```python
from build123d import *

# Parameters (mm, degrees)
SKETCH2_R                = 11.43
BOSS_EXTRUDE1_DEPTH      = 5.08
BOSS_EXTRUDE2_DEPTH      = 5.08
SKETCH4_R                = 4.318
SKETCH4_R_2              = 2.032
CUT_EXTRUDE1_DEPTH       = 5.08
CIRPATTERN1_COUNT        = 4
BOSS_EXTRUDE3_DEPTH      = 38.1
BOSS_EXTRUDE3_DEPTH_BACK = 40.64
SKETCH9_R                = 11.43
BOSS_EXTRUDE4_DEPTH      = 6.35


with BuildPart() as part:
    # Sketch2 → Boss-Extrude1 (new body)
    with BuildSketch(Plane.XY):
        Circle(SKETCH2_R)
    extrude(amount=BOSS_EXTRUDE1_DEPTH)

    # Sketch7 → Boss-Extrude2 (add)
    with BuildSketch(Plane(origin=(0, 0, 0), x_dir=(-1, 0, 0), z_dir=(0, 0, -1))):
        with BuildLine():
            Line((0, 11.43), (32.334928423, 11.43))
            ThreePointArc((32.334928423, 11.43), (43.764928423, 0), (32.334928423, -11.43))
            Line((32.334928423, -11.43), (0, -11.43))
            Line((0, -11.43), (0, 11.43))
        make_face()
    extrude(amount=-BOSS_EXTRUDE2_DEPTH)

    # Sketch4 → Cut-Extrude1 (cut)
    with BuildSketch(Plane(origin=(0, 0, 0), x_dir=(-1, 0, 0), z_dir=(0, 0, -1))):
        Circle(SKETCH4_R)
        with Locations((0, -8.001)):
            Circle(SKETCH4_R_2)
    cut_extrude1 = extrude(amount=-CUT_EXTRUDE1_DEPTH, mode=Mode.SUBTRACT)

    # CirPattern1: Cut-Extrude1 ×4 about axis
    cirpattern1_axis = Axis((0, 0, 0), (0, 0, 1))
    for i in range(1, CIRPATTERN1_COUNT):
        add(cut_extrude1.rotate(cirpattern1_axis, i * 360 / CIRPATTERN1_COUNT), mode=Mode.SUBTRACT)

    # Sketch9 → Boss-Extrude3 (add, two sides: drawn at the far end of the back side and taken through both)
    with BuildSketch(Plane.XY.offset(5.08).offset(-BOSS_EXTRUDE3_DEPTH_BACK)):
        with Locations((-32.334928423, 0)):
            Circle(SKETCH9_R)
    extrude(amount=BOSS_EXTRUDE3_DEPTH + BOSS_EXTRUDE3_DEPTH_BACK)

    # Sketch10 → Boss-Extrude4 (add)
    with BuildSketch(Plane.XY.offset(-31.75)):
        with BuildLine():
            Line((-37.028733454, -72.582202646), (-43.258278065, -30.219589225))
            Line((-43.258278065, -30.219589225), (-20.904928423, 0))
            Line((-20.904928423, 0), (-32.171436877, 0.015474968))
            Line((-32.171436877, 0.015474968), (-39.730825163, 0.025858069))
            Line((-39.730825163, 0.025858069), (-53.950343023, -30.219589225))
            Line((-53.950343023, -30.219589225), (-53.950343023, -58.308345581))
            Line((-53.950343023, -58.308345581), (-43.258278065, -84.842076202))
            Line((-43.258278065, -84.842076202), (-24.756596451, -88.874141931))
            ThreePointArc((-24.756596451, -88.874141931), (-19.207535115, -84.404142538), (-24.756596451, -79.934143145))
            Line((-24.756596451, -79.934143145), (-37.028733454, -72.582202646))
        make_face()
    boss_extrude4 = extrude(amount=BOSS_EXTRUDE4_DEPTH)

    # Mirror1: Boss-Extrude4 across plane
    add(boss_extrude4.mirror(Plane.XY))


solid = part.part
```
Read the model definition and answer for the solid it produces. Units are mm, in the model's axes. A direction names the side the tool comes from. Coordinates: 2 decimals unless noted, no trailing zeros. Loops run counter-clockwise (first coordinate to the right, second up) from the corner with the lowest first, then second, coordinate; pieces in that order, holes last.
(1) The mould has two halves that part along Z. Classify faces 3 (the face through (-19.21, -84.52, -28.62)), 4 (the face through (-41, -56, 31.75)), 5 (the face through (-41, -56, 25.4)): released by +Z, released by -Z, zero draft, split by the parting line, or undercut.
Solution:
face 3: zero draft
face 4: released by +Z
face 5: undercut
(2) The part is cut by section B-B (y = -26). Determine the outline of the cut face in (x, z), and give its area (3 significant figures).
Solution:
outline: (-51.97, -31.75) - (-40.14, -31.75) - (-40.14, -25.4) - (-51.97, -25.4) - close; (-51.97, 25.4) - (-40.14, 25.4) - (-40.14, 31.75) - (-51.97, 31.75) - close
area: 150 mm2
(3) The part is cut by section A-A (y = 0). Determine the outline of the cut face in (x, z).
Solution:
outline: (-43.76, -35.56) - (-20.9, -35.56) - (-20.9, 0) - (-10.03, 0) - (-10.03, 5.08) - (-20.9, 5.08) - (-20.9, 43.18) - (-43.76, 43.18) - close; (-5.97, 0) - (-4.32, 0) - (-4.32, 5.08) - (-5.97, 5.08) - close; (4.32, 0) - (5.97, 0) - (5.97, 5.08) - (4.32, 5.08) - close; (10.03, 0) - (11.43, 0) - (11.43, 5.08) - (10.03, 5.08) - close
(4) A tool of negligible diameter and unlimited length cuts with its end or side. For faces 1 (the face through (-40.1, -51.7, 28.6)), 2 (the face through (-34.14, -86.83, -28.62)), from which of +Z, -Z, +X, -X, +Y, -Y can it reach the whole face along a straight path? Write none if from no direction.
Solution:
face 1: +Z, -Z, +X
face 2: +Z, -Z, -X, -Y
(5) The part is cut by section D-D (x = -15). Determine the outline of the cut face in (y, z).
Solution:
outline: (-11.43, 0) - (11.43, 0) - (11.43, 5.08) - (-11.43, 5.08) - close
(6) Flat-ended cylindrical pins translate along their axes: pin 1 Ø11 at (x, y) = (0, 0) entering from -Z; pin 2 Ø6.5 at (x, y) = (8.001, 0) entering from +Z; pin 3 Ø17.5 at (x, y) = (-42, -31.5) entering from -Z. Find the tip coordinate at first contact, or state that the pin passes through.
Solution:
pin 1: stops at z = 0
pin 2: stops at z = 5.08
pin 3: stops at z = -31.75
(7) The part is cut by section C-C (z = 3.5). Determine the outline of the cut face in (x, y).
Solution:
outline: (-32.33, -11.43) - (0, -11.43) arc R11.43 ccw to (0, 11.43) - (-32.33, 11.43) arc R11.43 ccw to start; hole circle Ø4.06 at (-8, 0); hole circle Ø8.64 at (0, 0); hole circle Ø4.06 at (0, -8); hole circle Ø4.06 at (0, 8); hole circle Ø4.06 at (8, 0)
(8) Consider line 1 along Y through (x, z) = (0, 1); line 2 along Z through (x, y) = (-41, -73); line 3 along Y through (x, z) = (-37, 30.5). Determine where each line is inside the solid, lowest interval first.
Solution:
line 1: y = -11.43 to -10.03, -5.97 to -4.32, 4.32 to 5.97, 10.03 to 11.43
line 2: z = -31.75 to -25.4, 25.4 to 31.75
line 3: y = -86.21 to -72.6, -21.76 to 10.43
